Can you work these out from the model? Positions are in its coordinate system, mm. A direction names the side the tool comes from. Give positions to 0.01 mm unless a question says otherwise; leave off trailing zeros. Write each loop counter-clockwise with the first axis right and the second up, starting at its lowest first coordinate (ties: lowest second). Pieces come first, ordered by that corner, then holes. Notation, with made-up numbers: (62.5, 51.25) -> (97.5, 51.25) arc R15 ccw to (97.5, 61.25) -> close; hole circle Ø7 at (43.5, -35.75). An arc over 180 degrees is marked (long way). One line per item, written item: value.
from build123d import *

# Parameters (mm, degrees)
VOLUME_KNOB_R                      = 35
KNOB_TOP_DEPTH                     = 3.5
VOLUME_KNOB_3_R                    = 35
VOLUME_KNOB_3_R_2                  = 32
KNOB_WALLS_DEPTH                   = 26
KNOB_START                         = 3.5
KNOB_SHAFT_KEYWAY_DEPTH            = 10
VOLUME_KNOB_8_R                    = 29.33
VOLUME_KNOB_8_R_2                  = 3
KNOB_DAMEPNING_EXTENSION_TOP_DEPTH = 12.9
KNOB_START_2                       = 16.4
VOLUME_KNOB_11_R                   = 10
VOLUME_KNOB_11_R_2                 = 3
KNOB_SHAFT_SUPPORT_DEPTH           = 5


with BuildPart() as part:
    # Volume Knob → Knob Top (new body)
    with BuildSketch(Plane(origin=(0, 0, 0), x_dir=(1, 0, 0), z_dir=(0, 1, 0))):
        with Locations(Location((0, 0, 0), (0, 0, 270))):
            Circle(VOLUME_KNOB_R)
    extrude(amount=KNOB_TOP_DEPTH)

    # Volume Knob<3> → Knob Walls (add)
    with BuildSketch(Plane(origin=(0, 0, 0), x_dir=(1, 0, 0), z_dir=(0, 1, 0))):
        with Locations(Location((0, 0, 0), (0, 0, 270))):
            Circle(VOLUME_KNOB_3_R)
        with Locations(Location((0, 0, 0), (0, 0, 90))):
            Circle(VOLUME_KNOB_3_R_2, mode=Mode.SUBTRACT)
    extrude(amount=KNOB_WALLS_DEPTH)

    # Volume Knob<4> → Knob Shaft Keyway (add)
    with BuildSketch(Plane(origin=(0, 0, 0), x_dir=(1, 0, 0), z_dir=(0, 1, 0)).offset(KNOB_START)):
        with BuildLine():
            Line((-2.598076211, 1.5), (2.598076211, 1.5))
            ThreePointArc((2.598076211, 1.5), (0, 3), (-2.598076211, 1.5))
        make_face()
    extrude(amount=KNOB_SHAFT_KEYWAY_DEPTH)

    # Volume Knob<8> → Knob Damepning Extension (top) (add)
    with BuildSketch(Plane(origin=(0, 0, 0), x_dir=(1, 0, 0), z_dir=(0, 1, 0)).offset(KNOB_START)):
        with Locations(Location((0, 0, 0), (0, 0, 90))):
            Circle(VOLUME_KNOB_8_R)
        with Locations(Location((0, 0, 0), (0, 0, 150))):
            Circle(VOLUME_KNOB_8_R_2, mode=Mode.SUBTRACT)
    extrude(amount=KNOB_DAMEPNING_EXTENSION_TOP_DEPTH)

    # Volume Knob<11> → Knob Shaft Support (add)
    with BuildSketch(Plane(origin=(0, 0, 0), x_dir=(1, 0, 0), z_dir=(0, 1, 0)).offset(KNOB_START_2)):
        with Locations(Location((0, 0, 0), (0, 0, 270))):
            Circle(VOLUME_KNOB_11_R)
        with Locations(Location((0, 0, 0), (0, 0, 150))):
            Circle(VOLUME_KNOB_11_R_2, mode=Mode.SUBTRACT)
    extrude(amount=KNOB_SHAFT_SUPPORT_DEPTH)


solid = part.part
1) For faces 4 (the face through (0, 0, 0)), 5 (the face through (11.234, 9.86, -27.093)), which set-ups out of +Z, -Z, +X, -X, +Y, -Y let a thin tool reach every point of the face, with its end or its side?
Answer list:
face 4: +Z, -Z, +X, -X, -Y
face 5: +Y
2) If we section it at D-D (y = 23.5): Write out the boundary of the cut face in (x, z).
Answer list:
outline: circle Ø70 at (0, 0); hole circle Ø64 at (0, 0)
3) We'd pull the mould along Z, two halves only. Please class faces 1 (the face through (-21, 13, -28)), 2 (the face through (-28.4, 26, 15.4)), 3 (the face through (-26, 3.5, 14)): released by +Z, released by -Z, zero draft, split by the parting line, or undercut.
Answer list:
face 1: split by the parting line
face 2: zero draft
face 3: undercut
4) If we section it at C-C (x = 0): Write out the boundary of the cut face in (y, z), and give its area (3 significant figures).
Answer list:
outline: (0, -35) -> (26, -35) -> (26, -32) -> (3.5, -32) -> (3.5, -29.33) -> (16.4, -29.33) -> (16.4, -10) -> (21.4, -10) -> (21.4, -3) -> (13.5, -3) -> (13.5, -1.5) -> (3.5, -1.5) -> (3.5, 3) -> (21.4, 3) -> (21.4, 10) -> (16.4, 10) -> (16.4, 29.33) -> (3.5, 29.33) -> (3.5, 32) -> (26, 32) -> (26, 35) -> (0, 35) -> close
area: 1,140 mm^2
5) Will these pins go through, and if not, where does the flat tip stop? pin 1 (1 mm diameter, centred on x = 0.5, z = 8, fed in from +Y); pin 2 (8 mm diameter, centred on x = 12.5, y = 10, fed in from +Z); pin 3 (6 mm diameter, centred on y = 6.5, z = 26.5, fed in from -X).
Answer list:
pin 1: stops at y = 21.4
pin 2: stops at z = 33.95
pin 3: stops at x = -25.94
6) I need wall thicknesses on L1, parallel to X at y = 15, z = 0; L2, parallel to X at y = 20.5, z = 0; L3, parallel to Z at x = -5, y = 5.25. Which ranges of each line are inside material? Lowest first, please.
Answer list:
L1: x = -35 to -32, -29.33 to -3, 3 to 29.33, 32 to 35
L2: x = -35 to -32, -10 to -3, 3 to 10, 32 to 35
L3: z = -34.64 to -31.61, -28.9 to 28.9, 31.61 to 34.64
7) If we section it at A-A (y = 11.5): Write out the boundary of the cut face in (x, z), and give its area (3 significant figures).
Answer list:
outline: circle Ø70 at (0, 0); circle Ø58.66 at (0, 0); hole circle Ø64 at (0, 0); hole (-2.6, -1.5) -> (2.6, -1.5) arc R3 ccw (long way) to start
area: 3,310 mm^2
8) If we section it at B-B (z = 0): Write out the boundary of the cut face in (x, y), and give its area (3 significant figures).
Answer list:
outline: (-35, 0) -> (35, 0) -> (35, 26) -> (32, 26) -> (32, 3.5) -> (29.33, 3.5) -> (29.33, 16.4) -> (10, 16.4) -> (10, 21.4) -> (3, 21.4) -> (3, 3.5) -> (-3, 3.5) -> (-3, 21.4) -> (-10, 21.4) -> (-10, 16.4) -> (-29.33, 16.4) -> (-29.33, 3.5) -> (-32, 3.5) -> (-32, 26) -> (-35, 26) -> close
area: 1,130 mm^2
